from build123d import *

# Parameters (mm, degrees)
SKETCH_1_W          = 30
SKETCH_1_H          = 30
EXTRUDE_1_DEPTH     = 30
SKETCH_5_W          = 10
SKETCH_5_H          = 10
CUT_EXTRUDE_4_DEPTH = 52.961524227
SKETCH_7_W          = 20
SKETCH_7_H          = 10
CUT_EXTRUDE_5_DEPTH = 52.961524227
SKETCH_9_W          = 10
SKETCH_9_H          = 10
CUT_EXTRUDE_6_DEPTH = 52.961524227
SKETCH_10_W         = 10
SKETCH_10_H         = 10
CUT_EXTRUDE_7_DEPTH = 15


with BuildPart() as part:
    # 草圖1 → 填料-伸1 (new body)
    with BuildSketch(Plane.XY):
        with Locations((15, 15)):
            Rectangle(SKETCH_1_W, SKETCH_1_H)
    extrude(amount=-EXTRUDE_1_DEPTH)

    # 草圖5 → 除料-伸長4 (cut, through all)
    with BuildSketch(Plane.XY):
        with Locations((15, 25)):
            Rectangle(SKETCH_5_W, SKETCH_5_H)
    extrude(amount=-CUT_EXTRUDE_4_DEPTH, mode=Mode.SUBTRACT)

    # 草圖7 → 除料-伸長5 (cut, through all)
    with BuildSketch(Plane(origin=(0, 30, 0), x_dir=(1, 0, 0), z_dir=(0, 1, 0))):
        with Locations((20, 5)):
            Rectangle(SKETCH_7_W, SKETCH_7_H)
    extrude(amount=-CUT_EXTRUDE_5_DEPTH, mode=Mode.SUBTRACT)

    # 草圖9 → 除料-伸長6 (cut, through all)
    with BuildSketch(Plane(origin=(30, 0, 0), x_dir=(0, 0, -1), z_dir=(1, 0, 0))):
        with Locations((5, 25)):
            Rectangle(SKETCH_9_W, SKETCH_9_H)
    extrude(amount=-CUT_EXTRUDE_6_DEPTH, mode=Mode.SUBTRACT)

    # 草圖10 → 除料-伸長7 (cut)
    with BuildSketch(Plane(origin=(30, 0, 0), x_dir=(0, 0, -1), z_dir=(1, 0, 0))):
        with Locations((15, 25)):
            Rectangle(SKETCH_10_W, SKETCH_10_H)
    extrude(amount=-CUT_EXTRUDE_7_DEPTH, mode=Mode.SUBTRACT)


solid = part.part
For this review, take the finished solid that the model builds, in its own axes (mm). A direction names the side the tool comes from. Coordinates: 2 decimals unless noted, no trailing zeros. Order: outer loops, then holes, each group sorted by start corner. A loop starts at its lowest first (then second) coordinate and runs counter-clockwise, first axis right, second up. Notation, with made-up numbers: (-27.75, -13) -> (10.25, -13) arc R27 ccw to (10.25, 17) -> close; hole circle Ø2 at (22.5, 58). An arc over 180 degrees is marked (long way). Return JSON: item names as keys, results as strings.
1. We need section D-D on y = 3.5. Write out the cut boundary in (x, z), and give its area (3 significant figures).
Answer block:
{"outline": "(0, -30) -> (30, -30) -> (30, -10) -> (10, -10) -> (10, 0) -> (0, 0) -> close", "area": "700 mm²"}
2. We need section C-C on z = -21.5. Write out the cut boundary in (x, y), and give its area (3 significant figures).
Answer block:
{"outline": "(0, 0) -> (30, 0) -> (30, 30) -> (20, 30) -> (20, 20) -> (10, 20) -> (10, 30) -> (0, 30) -> close", "area": "800 mm²"}
3. We need section A-A on y = 20.5. Write out the cut boundary in (x, z).
Answer block:
{"outline": "(0, -30) -> (10, -30) -> (10, -10) -> (0, -10) -> close; (20, -30) -> (30, -30) -> (30, -20) -> (20, -20) -> close"}
4. The part is to be moulded in two halves that separate along X. For faces 4 (the flat face through (20, 10, -10)), 5 (the flat face through (30, 11, -20)), 6 (the flat face through (18, 20, -18)), say which applies: +X half, -X half, draft (parallel to the pull), parting line (faces both ways), or undercut.
Answer block:
{"face 4": "draft", "face 5": "+X half", "face 6": "undercut"}
5. For pin 1 Ø6 at (x, y) = (11, 24) entering from -Z; pin 2 Ø8 at (x, y) = (6, 25.5) entering from +Z; pin 3 Ø11 at (y, z) = (13, -3) entering from +X; pin 4 Ø5 at (x, z) = (7.5, -7) entering from +Y, all flat-tipped, find the tip position at first contact; note any pin that passes through.
Answer block:
{"pin 1": "z = -30", "pin 2": "z = -10", "pin 3": "x = 10", "pin 4": "y = 20"}
6. Machinability: for faces 1 (the flat face through (5, 25, -10)), 2 (the flat face through (10, 10, -5)), 3 (the flat face through (10, 25, -20)), which of the approach directions +Z, -Z, +X, -X, +Y, -Y give a long, thin tool a straight path to every point of the face, cutting with its end or side? Answer none if there is none.
Answer block:
{"face 1": "+Z, +X, -X, +Y", "face 2": "+Z, +X, +Y, -Y", "face 3": "+Z, -Z, +Y"}
7. We need section B-B on x = 22. Write out the cut boundary in (y, z), and give its area (3 significant figures).
Answer block:
{"outline": "(0, -30) -> (30, -30) -> (30, -20) -> (20, -20) -> (20, -10) -> (0, -10) -> close", "area": "500 mm²"}
8. For line 1 (X direction, y = 23.75, z = -20.25); line 2 (Z direction, x = 16.25, y = 14.25); line 3 (X direction, y = 16, z = -7.5), list the stretches that pass through material, from the lowest coordinate up. Write a range as from..to.
Answer block:
{"line 1": "0..10, 20..30", "line 2": "-30..-10", "line 3": "0..10"}
